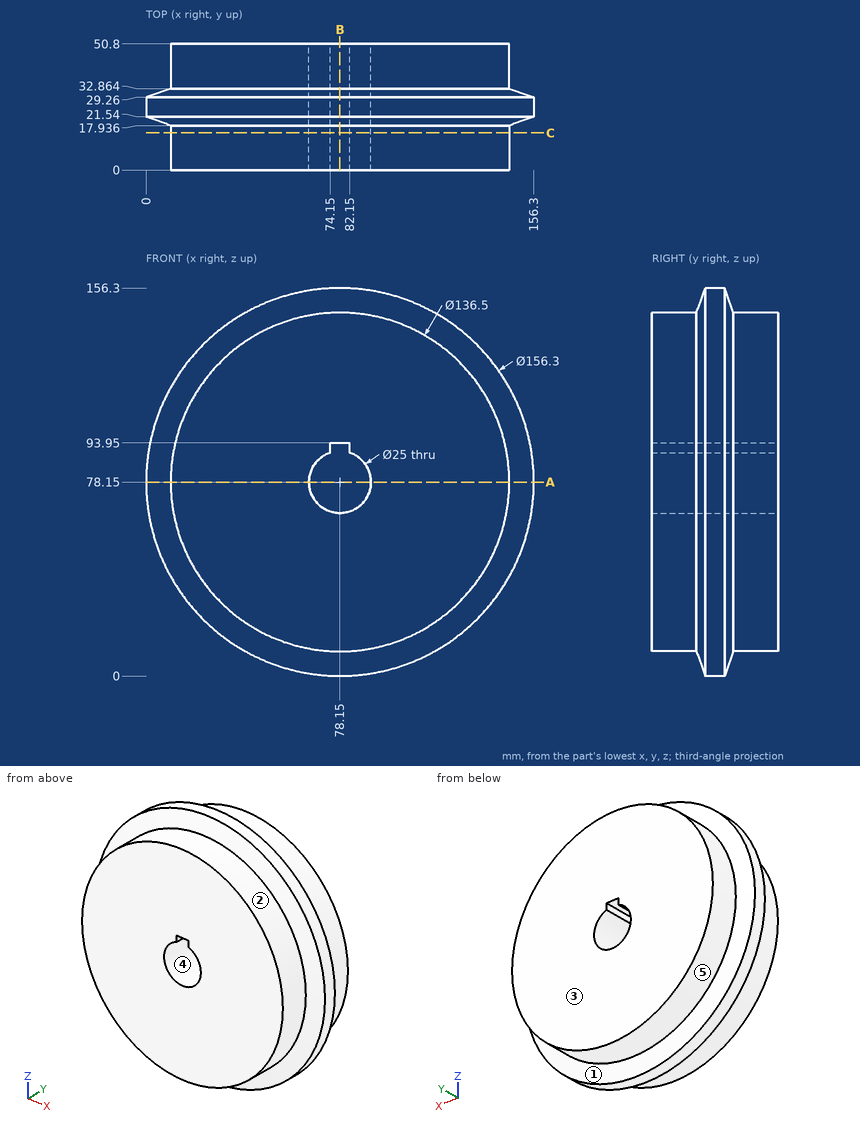
Geometry check sheet. Reference: drawing and pictorial views, mm from the part's lowest x, y, z. A direction names the side the tool comes from. Coordinates: 2 decimals unless noted, no trailing zeros. Order: outer loops, then holes, each group sorted by start corner. A loop starts at its lowest first (then second) coordinate and runs counter-clockwise, first axis right, second up. Notation, with made-up numbers: (32, -16.75) -> (71, -16.75) arc R32 ccw to (71, 18.25) -> close; hole circle Ø10 at (53, -33.5). An arc over 180 degrees is marked (long way). Put each result on its own line as item: value. Start each with the question number.
1) Cross-section at B-B (x = 78.15). Enter the section's corners in (y, z).
2) Cross-section at C-C (y = 15). Enter the section's corners in (x, z), plus the area to 3 significant figures.
3) Tool access check on the marked faces 1 and 2. Record the directions out of +Z, -Z, +X, -X, +Y, -Y that give a thin tool (end or side, any length) a straight path to the whole face; none if there is none.
4) Material ranges on L1, parallel to Z at x = 78.15, y = 13; L2, parallel to Z at x = 78.15, y = 25; L3, parallel to X at y = 22, z = 78, recorded low to high.
5) Release check for a two-part mould opening along X. For the marked faces 3, 4 and 5 record: pulls with the +X half, pulls with the -X half, needs draft (parallel to the pull), parting line crosses it, or undercut.
6) Go/stop test with flat-tipped pins: pin 1 (2 mm diameter, centred on x = 129.5, y = 28, fed in from -Z); pin 2 (5 mm diameter, centred on x = 82, y = 27.5, fed in from -Z); pin 3 (12 mm diameter, centred on x = 132, y = 27.5, fed in from -Z). Record where each tip stops, or that it passes through.
7) Cross-section at A-A (z = 78.15). Enter the section's corners in (x, y), plus the area to 3 significant figures.
Geometry check:
1. outline: (0, 9.9) -> (17.94, 9.9) -> (21.54, 0) -> (29.26, 0) -> (32.86, 9.9) -> (50.8, 9.9) -> (50.8, 65.65) -> (0, 65.65) -> close; (0, 93.95) -> (50.8, 93.95) -> (50.8, 146.4) -> (32.86, 146.4) -> (29.26, 156.3) -> (21.54, 156.3) -> (17.94, 146.4) -> (0, 146.4) -> close
2. outline: circle Ø136.5 at (78.15, 78.15); hole (74.15, 89.99) arc R12.5 ccw (long way) to (82.15, 89.99) -> (82.15, 93.95) -> (74.15, 93.95) -> close
2. area: 14,100 mm^2
3. face 1: +Y
3. face 2: -Y
4. L1: z = 9.9 to 65.65, 93.95 to 146.4
4. L2: z = 0 to 65.65, 93.95 to 156.3
4. L3: x = 0 to 65.65, 90.65 to 156.3
5. face 3: needs draft
5. face 4: undercut
5. face 5: parting line crosses it
6. pin 1: stops at z = 18.38
6. pin 2: stops at z = 0.01
6. pin 3: stops at z = 16.36
7. outline: (0, 21.54) -> (9.9, 17.94) -> (9.9, 0) -> (65.65, 0) -> (65.65, 50.8) -> (9.9, 50.8) -> (9.9, 32.86) -> (0, 29.26) -> close; (90.65, 0) -> (146.4, 0) -> (146.4, 17.94) -> (156.3, 21.54) -> (156.3, 29.26) -> (146.4, 32.86) -> (146.4, 50.8) -> (90.65, 50.8) -> close
7. area: 5,890 mm^2
